```python
from build123d import *

# Parameters (mm, degrees)
F0_W       = 7
F0_H       = 6
F1_DEPTH   = 3.5
F2_DEPTH   = 15
F3_W       = 55.5
F3_H       = 9.5
F4_DEPTH   = 100
F3_W_2     = 53.1
F3_H_2     = 2.1
F5_DEPTH   = 48.65
F6_SIZE2   = 1
F6_SIZE    = 2
F6_2_SIZE2 = 1
F6_2_SIZE  = 2
F6_3_SIZE2 = 1
F6_3_SIZE  = 2
F7_SIZE2   = 2
F7_SIZE    = 1
F8_R       = 2


with BuildPart() as f1:
    # F0 (on Top) → F1 (new body)
    with BuildSketch(Plane.XY):
        with Locations((-59, 43)):
            Rectangle(F0_W, F0_H)
        with BuildLine():
            add(Edge.make_bspline(
                [(-55.5, 46), (-35.0651084215, 46.3366690111), (-13.1863134629, 47.1130676767), (3.5, 36)],
                knots=[0, 0, 0, 0, 0.4365224183, 0.4365224183, 0.4365224183, 0.4365224183], degree=3))
            Line((-55.5, 46), (-55.5, 40))
            add(Edge.make_bspline(
                [(-55.5, 40), (-37.1709838309, 40.05441996), (-18.4495575403, 40.3060604222), (-3.5, 30)],
                knots=[0, 0, 0, 0, 0.4215444213, 0.4215444213, 0.4215444213, 0.4215444213], degree=3))
            Line((-3.5, 30), (-3.5, 36))
            Line((-3.5, 36), (3.5, 36))
        make_face()
        with Locations((0, 33)):
            Rectangle(F0_W, F0_H)
        with BuildLine():
            add(Edge.make_bspline(
                [(3.5, 36), (12.561299992, 29.9651834856), (20.0913884934, 20.4242808164), (27.3811387561, 8.8639486742)],
                knots=[0.4365224183, 0.4365224183, 0.4365224183, 0.4365224183, 0.6735706191, 0.6735706191, 0.6735706191, 0.6735706191], degree=3))
            Line((3.5, 36), (3.5, 30))
            Line((3.5, 30), (-3.5, 30))
            add(Edge.make_bspline(
                [(-3.5, 30), (5.9722353572, 23.4699452033), (13.930195357, 12.7013372284), (21.9258388158, -0.3794873482)],
                knots=[0.4215444213, 0.4215444213, 0.4215444213, 0.4215444213, 0.688640485, 0.688640485, 0.688640485, 0.688640485], degree=3))
            add(Edge.make_bspline(
                [(21.9258388158, -0.3794873482), (23.7468548988, 2.5891115783), (25.5585039934, 5.6780700829), (27.3811387561, 8.8639486742)],
                knots=[0.6903483348, 0.6903483348, 0.6903483348, 0.6903483348, 0.7497888406, 0.7497888406, 0.7497888406, 0.7497888406], degree=3))
        make_face()
        with BuildLine():
            add(Edge.make_bspline(
                [(27.3811387561, 8.8639486742), (29.1720644783, 6.0238381842), (30.9484840318, 3.0618403714), (32.7295390228, 0)],
                knots=[0.6735706191, 0.6735706191, 0.6735706191, 0.6735706191, 0.7318079668, 0.7318079668, 0.7318079668, 0.7318079668], degree=3))
            add(Edge.make_bspline(
                [(21.9258388158, -0.3794873482), (23.7468548988, 2.5891115783), (25.5585039934, 5.6780700829), (27.3811387561, 8.8639486742)],
                knots=[0.6903483348, 0.6903483348, 0.6903483348, 0.6903483348, 0.7497888406, 0.7497888406, 0.7497888406, 0.7497888406], degree=3))
            add(Edge.make_bspline(
                [(21.9258388158, -0.3794873482), (23.6633015374, -3.221965904), (25.4025436645, -6.1736268671), (27.1594897195, -9.2147042555)],
                knots=[0.688640485, 0.688640485, 0.688640485, 0.688640485, 0.7466807736, 0.7466807736, 0.7466807736, 0.7466807736], degree=3))
            add(Edge.make_bspline(
                [(27.1594897195, -9.2147042555), (29.0255530458, -6.267974343), (30.875033208, -3.1881108676), (32.7295390228, 0)],
                knots=[0.6711689071, 0.6711689071, 0.6711689071, 0.6711689071, 0.7318079668, 0.7318079668, 0.7318079668, 0.7318079668], degree=3))
        make_face()
        with BuildLine():
            add(Edge.make_bspline(
                [(27.3811387561, 8.8639486742), (35.0534078745, 22.2747089818), (42.9203361457, 37.4028324845), (52.5, 52.5)],
                knots=[0.7497888406, 0.7497888406, 0.7497888406, 0.7497888406, 1, 1, 1, 1], degree=3))
            add(Edge.make_bspline(
                [(27.3811387561, 8.8639486742), (29.1720644783, 6.0238381842), (30.9484840318, 3.0618403714), (32.7295390228, 0)],
                knots=[0.6735706191, 0.6735706191, 0.6735706191, 0.6735706191, 0.7318079668, 0.7318079668, 0.7318079668, 0.7318079668], degree=3))
            add(Edge.make_bspline(
                [(32.7295390228, 0), (40.9315739468, 14.1002505736), (49.2319147047, 30.3179077966), (59.5, 46.5)],
                knots=[0.7318079668, 0.7318079668, 0.7318079668, 0.7318079668, 1, 1, 1, 1], degree=3))
            Line((59.5, 46.5), (52.5, 46.5))
            Line((52.5, 46.5), (52.5, 52.5))
        make_face()
        with BuildLine():
            add(Edge.make_bspline(
                [(32.7295390228, 0), (40.9315739468, -14.1002505736), (49.2319147047, -30.3179077966), (59.5, -46.5)],
                knots=[0.7318079668, 0.7318079668, 0.7318079668, 0.7318079668, 1, 1, 1, 1], degree=3))
            add(Edge.make_bspline(
                [(27.1594897195, -9.2147042555), (29.0255530458, -6.267974343), (30.875033208, -3.1881108676), (32.7295390228, 0)],
                knots=[0.6711689071, 0.6711689071, 0.6711689071, 0.6711689071, 0.7318079668, 0.7318079668, 0.7318079668, 0.7318079668], degree=3))
            add(Edge.make_bspline(
                [(27.1594897195, -9.2147042555), (34.8277530321, -22.4876115835), (42.833262349, -37.4638320009), (52.5, -52.5)],
                knots=[0.7466807736, 0.7466807736, 0.7466807736, 0.7466807736, 1, 1, 1, 1], degree=3))
            Line((52.5, -52.5), (52.5, -46.5))
            Line((52.5, -46.5), (59.5, -46.5))
        make_face()
        with BuildLine():
            add(Edge.make_bspline(
                [(21.9258388158, -0.3794873482), (23.6633015374, -3.221965904), (25.4025436645, -6.1736268671), (27.1594897195, -9.2147042555)],
                knots=[0.688640485, 0.688640485, 0.688640485, 0.688640485, 0.7466807736, 0.7466807736, 0.7466807736, 0.7466807736], degree=3))
            add(Edge.make_bspline(
                [(-3.5, -30), (6.2026375516, -23.5380533277), (14.1496419293, -13.0561517363), (21.9258388158, -0.3794873482)],
                knots=[0.4365224183, 0.4365224183, 0.4365224183, 0.4365224183, 0.6903483348, 0.6903483348, 0.6903483348, 0.6903483348], degree=3))
            Line((-3.5, -30), (3.5, -30))
            Line((3.5, -30), (3.5, -36))
            add(Edge.make_bspline(
                [(3.5, -36), (12.4694932079, -30.0263267098), (19.9386454326, -20.6172529014), (27.1594897195, -9.2147042555)],
                knots=[0.4365224183, 0.4365224183, 0.4365224183, 0.4365224183, 0.6711689071, 0.6711689071, 0.6711689071, 0.6711689071], degree=3))
        make_face()
        with Locations((56, 49.5)):
            Rectangle(F0_W, F0_H)
        with Locations((56, -49.5)):
            Rectangle(F0_W, F0_H)
        with Locations((0, -33)):
            Rectangle(F0_W, F0_H)
        with BuildLine():
            Line((-3.5, -36), (-3.5, -30))
            add(Edge.make_bspline(
                [(-55.5, -40.1135468303), (-37.1683816557, -40.3598255975), (-18.293541152, -39.8524832562), (-3.5, -30)],
                knots=[0.0495158831, 0.0495158831, 0.0495158831, 0.0495158831, 0.4365224183, 0.4365224183, 0.4365224183, 0.4365224183], degree=3))
            Line((-55.5, -40.1135468303), (-55.5, -46))
            add(Edge.make_bspline(
                [(-55.5, -46), (-35.0651084215, -46.3366690111), (-13.1863134629, -47.1130676767), (3.5, -36)],
                knots=[0, 0, 0, 0, 0.4365224183, 0.4365224183, 0.4365224183, 0.4365224183], degree=3))
            Line((3.5, -36), (-3.5, -36))
        make_face()
        with BuildLine():
            Line((-55.5, -46), (-55.5, -40.1135468303))
            add(Edge.make_bspline(
                [(-62.5, -40), (-60.1820166395, -40.0381892491), (-57.8454546318, -40.0820364822), (-55.5, -40.1135468303)],
                knots=[0, 0, 0, 0, 0.0495158831, 0.0495158831, 0.0495158831, 0.0495158831], degree=3))
            Line((-62.5, -40), (-62.5, -46))
            Line((-62.5, -46), (-55.5, -46))
        make_face()
    extrude(amount=F1_DEPTH)

    # F0 (on Top) → F2 (join)
    with BuildSketch(Plane.XY):
        with Locations((-59, 43)):
            Rectangle(F0_W, F0_H)
        with Locations((0, 33)):
            Rectangle(F0_W, F0_H)
        with BuildLine():
            Line((-55.5, -46), (-55.5, -40.1135468303))
            add(Edge.make_bspline(
                [(-62.5, -40), (-60.1820166395, -40.0381892491), (-57.8454546318, -40.0820364822), (-55.5, -40.1135468303)],
                knots=[0, 0, 0, 0, 0.0495158831, 0.0495158831, 0.0495158831, 0.0495158831], degree=3))
            Line((-62.5, -40), (-62.5, -46))
            Line((-62.5, -46), (-55.5, -46))
        make_face()
        with Locations((0, -33)):
            Rectangle(F0_W, F0_H)
        with Locations((56, 49.5)):
            Rectangle(F0_W, F0_H)
        with Locations((56, -49.5)):
            Rectangle(F0_W, F0_H)
    extrude(amount=F2_DEPTH)

    # F3 (on Front) → F4 (cut, symmetric)
    with BuildSketch(Plane.XZ):
        with Locations((-29.75, 8.25)):
            Rectangle(F3_W, F3_H)
    extrude(amount=F4_DEPTH, both=True, mode=Mode.SUBTRACT)

    # F3 (on Front) → F5 (cut, symmetric)
    with BuildSketch(Plane.XZ):
        with Locations((28.55, 8.05)):
            Rectangle(F3_W_2, F3_H_2)
    extrude(amount=F5_DEPTH, both=True, mode=Mode.SUBTRACT)

    # F6
    f6_edges = [f1.edges().sort_by_distance(p)[0] for p in [
        (-3.5, 33, 15),
    ]]
    f6_side = f1.faces().sort_by_distance((0, 33, 15))[0]
    chamfer(f6_edges, length=F6_SIZE, length2=F6_SIZE2, reference=f6_side)

    # F6#2
    f6_2_edges = [f1.edges().sort_by_distance(p)[0] for p in [
        (-3.5, -33, 15),
    ]]
    f6_2_side = f1.faces().sort_by_distance((0, -33, 15))[0]
    chamfer(f6_2_edges, length=F6_2_SIZE, length2=F6_2_SIZE2, reference=f6_2_side)

    # F6#3
    f6_3_edges = [f1.edges().sort_by_distance(p)[0] for p in [
        (-55.5, -43.056773, 15),
    ]]
    f6_3_side = f1.faces().sort_by_distance((-59.011322, -43.029185, 15))[0]
    chamfer(f6_3_edges, length=F6_3_SIZE, length2=F6_3_SIZE2, reference=f6_3_side)

    # F7
    f7_edges = [f1.edges().sort_by_distance(p)[0] for p in [
        (-55.5, 43, 15),
    ]]
    f7_side = f1.faces().sort_by_distance((-55.5, 43, 14))[0]
    chamfer(f7_edges, length=F7_SIZE, length2=F7_SIZE2, reference=f7_side)

    # F8
    f8_edges = [f1.edges().sort_by_distance(p)[0] for p in [
        (59.5, 52.5, 7.5),
        (59.5, -52.5, 7.5),
        (-62.5, -46, 7.5),
        (-62.5, 46, 7.5),
    ]]
    fillet(f8_edges, radius=F8_R)


solid = f1.part
```
Source: CAD feature listing. Evaluate the final solid. Frame: model axes, mm. A direction names the side the tool comes from. Give positions to 0.01 mm unless a question says otherwise; leave off trailing zeros.
(1) Access query for faces 1 (the face through (-59, -46, 7)), 2 (the face through (-2, -33, 8)), 3 (the face through (-57.5, -43, 8)), 4 (the face through (52.5, 49, 9)), 5 (the face through (1, -30, 9)). Directions: +Z, -Z, +X, -X, +Y, -Y. A direction counts if a zero-diameter tool reaches every point of the face in a straight line with its end or side. Return the directions, or none.
(2) Material intervals for line 1 along Z through (x, y) = (51, 35); line 2 along Y through (x, z) = (-23, 1.25); line 3 along X through (y, z) = (42, 9.75), sorted ascending.
(3) Contact query for flat-ended pins moving along their axis: P1, Ø2, axis at x = 0, z = 9, coming from the -Y side; P2, Ø5.5, axis at x = -59, z = 9.5, coming from the -Y side; P3, Ø3, axis at y = 32.5, z = 4.5, coming from the +X side. Output: stop coordinate, or through.
(4) Pull-direction query (Y, two-part tool) for faces 6 (the face through (55, -52.5, 7)), 7 (the face through (-60, 40, 7)), 8 (the face through (3.5, 33, 5)); classes: +Y half, -Y half, draft (parallel to the pull), parting line (faces both ways), or undercut.
Outcome:
1. face 1: +Z, -Z, -X, -Y
1. face 2: -X, +Y, -Y
1. face 3: +X, +Y, -Y
1. face 4: +Z, -X, +Y, -Y
1. face 5: +Z, +X, -X
2. line 1: z = 0 to 3.5
2. line 2: y = -45.1 to -37.91, 37.99 to 45.1
2. line 3: x = -62.5 to -57.5
3. P1: stops at y = -36
3. P2: stops at y = -46
3. P3: stops at x = 51.69
4. face 6: -Y half
4. face 7: undercut
4. face 8: draft
